Job drawing, mm, ordinate dimensions from the low corner. One solid piece. A direction names the side the tool comes from. Round coordinates to 2 decimals unless told otherwise and drop trailing zeros. Loops run counter-clockwise (first coordinate to the right, second up) from the corner with the lowest first, then second, coordinate; pieces in that order, holes last. Notation, with made-up numbers: M -20,15 L -1,15 A12 cw -1,32 Z; hole C 36,-28 d6. An arc over 180 degrees is marked long. One line per item, written item: value.
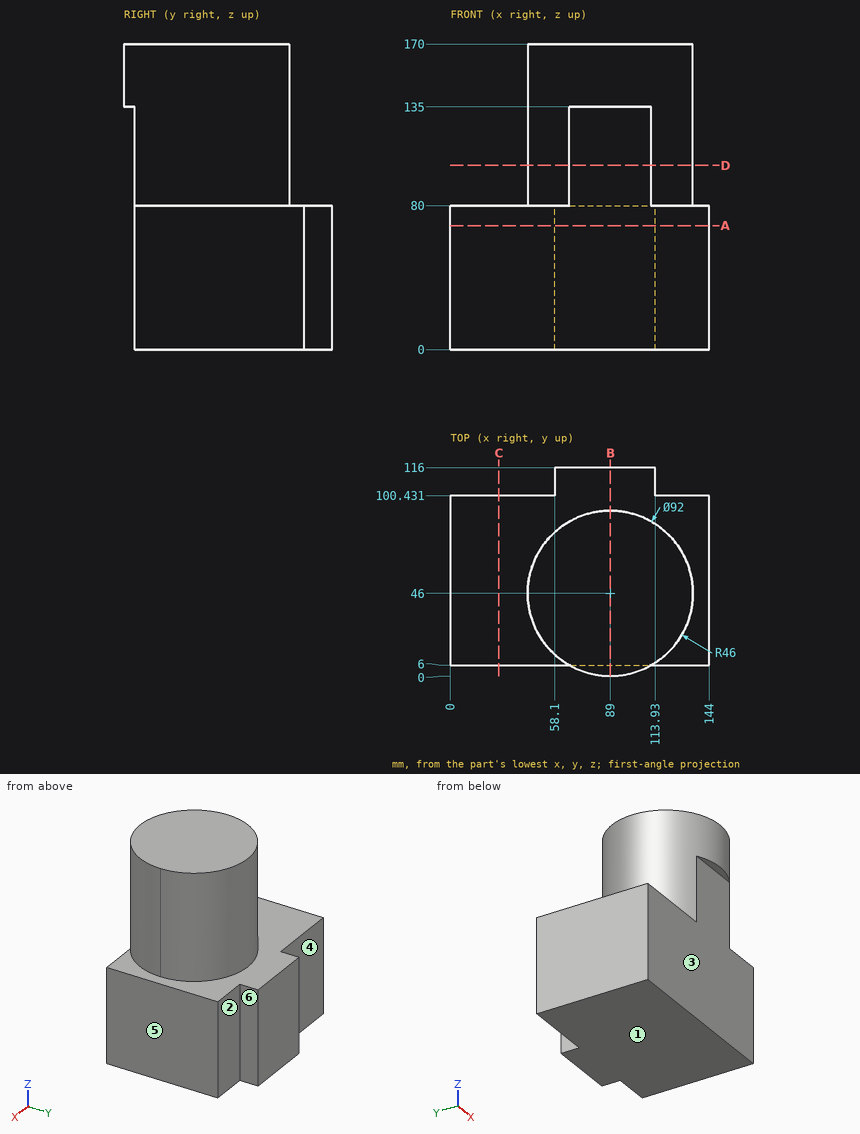
Item 1: Which spindle directions (+Z, -Z, +X, -X, +Y, -Y) get a long thin tool onto all of the face, cutting with end or side? Do the marked faces 4, 5 and 6. Say none if no direction does.
Check values:
face 4: +Z, -Z, -X, +Y
face 5: +Z, -Z, +X, +Y, -Y
face 6: +Z, -Z, +X, +Y
Item 2: Slice it at B-B, the plane x = 89. Give the cut face in (y, z).
Check values:
outline: M 0,135 L 6,135 L 6,0 L 116,0 L 116,80 L 92,80 L 92,170 L 0,170 Z
Item 3: Drop flat-ended pins along their axis: P1, Ø6, axis at x = 125.5, y = 46, coming from the -Z side; P2, Ø6, axis at x = 35, y = 81.5, coming from the +Z side; P3, Ø12.5, axis at y = 111, z = 58, coming from the -X side; P4, Ø1, axis at x = 86, z = 151.5, coming from the -Y side. Give the stop position or say it passes through.
Check values:
P1: stops at z = 0
P2: stops at z = 80
P3: stops at x = 58.1
P4: stops at y = 0.07
Item 4: Slice it at C-C, the plane x = 27. Give the cut face in (y, z), and give its area (3 significant figures).
Check values:
outline: M 6,0 L 100.43,0 L 100.43,80 L 6,80 Z
area: 7,550 mm2
Item 5: Slice it at D-D, the plane z = 102.5. Give the cut face in (x, y) (1 decimal).
Check values:
outline: M 66.3,6 L 111.7,6 A46 ccw long Z
Item 6: Pull direction Y, two halves, no side cores. Call the marked faces 1, 2 and 3: pulls with the +Y half, pulls with the -Y half, needs draft (parallel to the pull), parting line crosses it, or undercut.
Check values:
face 1: needs draft
face 2: pulls with the +Y half
face 3: pulls with the -Y half
Item 7: Slice it at A-A, the plane z = 69. Give the cut face in (x, y).
Check values:
outline: M 0,6 L 144,6 L 144,100.43 L 113.93,100.43 L 113.93,116 L 58.1,116 L 58.1,100.43 L 0,100.43 Z
Item 8: Wall check: line 1 along Z through (x, y) = (22.5, 52); line 2 along Y through (x, z) = (84, 9); line 3 along Y through (x, z) = (27.5, 78.5). Give the ranges that are in metal, low to high.
Check values:
line 1: z = 0 to 80
line 2: y = 6 to 116
line 3: y = 6 to 100.43
